Can you work these out from the model? Positions are in its coordinate system, mm. A direction names the side the tool comes from. Coordinates: 2 decimals unless noted, no trailing zeros. Write each loop counter-clockwise with the first axis right and the second up, starting at its lowest first coordinate (ties: lowest second). Pieces come first, ordered by that corner, then holes. Notation, with made-up numbers: (-25, 57.5) - (25, 57.5) arc R25 cw to (25, 71.5) - close; hole circle Ø1 at (40.5, 58). An arc over 180 degrees is marked (long way). One line per question, with ' | ' between items. Start each with the question number.
from build123d import *

# Parameters (mm, degrees)
EXTRUDE_THIN1_DEPTH     = 3
FILLET1_R               = 2
FILLET1_OF_MIRROR1_R    = 2
CIRPATTERN1_COUNT       = 2
CIRPATTERN1_ANGLE       = 90
CUT_EXTRUDE1_DEPTH      = 30.075421318
CUT_EXTRUDE1_DEPTH_BACK = 30.075421318
SKETCH3_R               = 1.625
CUT_EXTRUDE2_DEPTH      = 29.972057656
CUT_EXTRUDE2_DEPTH_BACK = 29.972057656
SKETCH4_R               = 1.5
FILLET2_R               = 8
CUT_EXTRUDE3_DEPTH      = 30.075421318
CUT_EXTRUDE3_DEPTH_BACK = 30.075421318
SKETCH5_R               = 5.5


with BuildPart() as part:
    # Sketch1 → Extrude-Thin1 (new, symmetric)
    with BuildSketch(Plane.XY):
        with BuildLine():
            Line((-20.409925586, -3), (-15.110133124, -3))
            ThreePointArc((-15.110133124, -3), (-14.249768469, -2.728728066), (-13.700594193, -2.013030215))
            Line((-13.700594193, -2.013030215), (-13.269638772, -0.828989928))
            ThreePointArc((-13.269638772, -0.828989928), (-13.08658068, -0.590423978), (-12.799792462, -0.5))
            Line((-12.799792462, -0.5), (0, -0.5))
            Line((0, -0.5), (0, 0.5))
            Line((0, 0.5), (-12.799792462, 0.5))
            ThreePointArc((-12.799792462, 0.5), (-13.660157116, 0.228728066), (-14.209331393, -0.486969785))
            Line((-14.209331393, -0.486969785), (-14.640286813, -1.671010072))
            ThreePointArc((-14.640286813, -1.671010072), (-14.823344906, -1.909576022), (-15.110133124, -2))
            Line((-15.110133124, -2), (-20.409925586, -2))
            Line((-20.409925586, -2), (-20.409925586, -3))
        make_face()
    extrude_thin1 = extrude(amount=EXTRUDE_THIN1_DEPTH, both=True)

    # Fillet1
    fillet1_edges = [part.edges().sort_by_distance(p)[0] for p in [
        (-20.409925586, -2.5, -3),
        (-20.409925586, -2.5, 3),
    ]]
    fillet(fillet1_edges, radius=FILLET1_R)

    # Mirror1: Extrude-Thin1 across plane
    add(extrude_thin1.mirror(Plane(origin=(0, 0.5, 3), x_dir=(0, 0, 1), z_dir=(1, 0, 0))))

    # Fillet1 of Mirror1
    fillet1_of_mirror1_edges = [part.edges().sort_by_distance(p)[0] for p in [
        (20.409925586, -2.5, -3),
        (20.409925586, -2.5, 3),
    ]]
    fillet(fillet1_of_mirror1_edges, radius=FILLET1_OF_MIRROR1_R)


with BuildPart() as cirpattern1_1:
    # CirPattern1: pattern copy
    add(part.part.rotate(Axis((0, 0, 0), (0, 1, 0)), 1 * CIRPATTERN1_ANGLE / (CIRPATTERN1_COUNT - 1)))


with BuildPart() as cut_extrude1_tool:
    # Sketch3 → Cut-Extrude1 (new, two sides: drawn at the far end of the back side and taken through both)
    with BuildSketch(Plane(origin=(0, 0.5, 0), x_dir=(1, 0, 0), z_dir=(0, 1, 0)).offset(-CUT_EXTRUDE1_DEPTH_BACK)):
        with Locations(Location((11.005, 0, 0), (0, 0, 270))):
            Circle(SKETCH3_R)
        with Locations(Location((0, -11.005, 0), (0, 0, 270))):
            Circle(SKETCH3_R)
        with Locations(Location((-11.005, 0, 0), (0, 0, 270))):
            Circle(SKETCH3_R)
        with Locations(Location((0, 11.005, 0), (0, 0, 270))):
            Circle(SKETCH3_R)
    extrude(amount=CUT_EXTRUDE1_DEPTH + CUT_EXTRUDE1_DEPTH_BACK)


with BuildPart() as part_1:
    add(part.part)

    # Cut-Extrude1: cut by cut_extrude1_tool
    add(cut_extrude1_tool.part, mode=Mode.SUBTRACT)


with BuildPart() as cirpattern1_1_1:
    add(cirpattern1_1.part)

    # Cut-Extrude1: cut by cut_extrude1_tool
    add(cut_extrude1_tool.part, mode=Mode.SUBTRACT)


with BuildPart() as cut_extrude2_tool:
    # Sketch4 → Cut-Extrude2 (new, two sides: drawn at the far end of the back side and taken through both)
    with BuildSketch(Plane(origin=(0, -2, 0), x_dir=(1, 0, 0), z_dir=(0, 1, 0)).offset(-CUT_EXTRUDE2_DEPTH_BACK)):
        with Locations(Location((-17.5, 0, 0), (0, 0, 180))):
            Circle(SKETCH4_R)
        with Locations(Location((0, 17.5, 0), (0, 0, 180))):
            Circle(SKETCH4_R)
        with Locations(Location((17.5, 0, 0), (0, 0, 180))):
            Circle(SKETCH4_R)
        with Locations(Location((0, -17.5, 0), (0, 0, 180))):
            Circle(SKETCH4_R)
    extrude(amount=CUT_EXTRUDE2_DEPTH + CUT_EXTRUDE2_DEPTH_BACK)


with BuildPart() as part_2:
    add(part_1.part)

    # Cut-Extrude2: cut by cut_extrude2_tool
    add(cut_extrude2_tool.part, mode=Mode.SUBTRACT)


with BuildPart() as cirpattern1_1_2:
    add(cirpattern1_1_1.part)

    # Cut-Extrude2: cut by cut_extrude2_tool
    add(cut_extrude2_tool.part, mode=Mode.SUBTRACT)


with BuildPart() as part_3:
    add(part_2.part)

    # Combine2: union CirPattern1_1
    add(cirpattern1_1_2.part)

    # Fillet2
    fillet2_edges = [part_3.edges().sort_by_distance(p)[0] for p in [
        (-3, 0, -3),
        (3, 0, -3),
        (-3, 0, 3),
        (3, 0, 3),
    ]]
    fillet(fillet2_edges, radius=FILLET2_R)

    # Sketch5 → Cut-Extrude3 (cut, two sides: drawn at the far end of the back side and taken through both)
    with BuildSketch(Plane(origin=(0, 0.5, 0), x_dir=(1, 0, 0), z_dir=(0, 1, 0)).offset(-CUT_EXTRUDE3_DEPTH_BACK)):
        with Locations(Location((0, 0, 0), (0, 0, 270))):
            Circle(SKETCH5_R)
    extrude(amount=CUT_EXTRUDE3_DEPTH + CUT_EXTRUDE3_DEPTH_BACK, mode=Mode.SUBTRACT)


solid = part_3.part
(1) If we section it at B-B on y = -2.5: List the corners of the cut face in (x, z) for me, plus the area to 3 significant figures.
(2) If we section it at D-D on x = 0: Give the number of separate pieces and of enclosed holes in the cut face, plus the area to 3 significant figures.
(3) I'm going to push flat-ended pins straight in: pin 1 (1 mm diameter, centred on y = -0.5, z = 10.5, fed in from +X); pin 2 (4 mm diameter, centred on x = 11.005, z = 0, fed in from +Y); pin 3 (6.5 mm diameter, centred on x = 0, z = 0, fed in from +Y); pin 4 (13 mm diameter, centred on x = -1, z = 4, fed in from -Y). Where does each tip first touch, or does it pass through?
(4) If I drill on probe 1 along Z at (x, y) = (17.5, -2.8); probe 2 along X at (y, z) = (-2.75, 0); probe 3 along X at (y, z) = (-0.3, 0), over which ranges is the centre line in solid material (lowest first)?
(5) If we mould it in two halves opening along X, with no side actions, what happens to faces 4 (the face through (-14.65, -2, -3)), 5 (the face through (-5.406, 0.007, 5.281)), 6 (the face through (13.49, -1.43, 0.04)), 7 (the face through (0.488, -0.007, 12.555))? For each: +X half, -X half, draft (parallel to the pull), parting line (faces both ways), or undercut.
(6) Which directions (+Z, -Z, +X, -X, +Y, -Y) give clear straight access to the entire face, cutting with the end or side of a thin tool? Please do faces 1 (the face through (14, -2, -3)), 2 (the face through (0.04, -1.43, 13.49)), 3 (the face through (-14.26, -2.736, 0.042)).
(7) If we section it at A-A on x = -17.5: List the corners of the cut face in (y, z) for me, plus the area to 3 significant figures.
(8) If we section it at C-C on z = 17.5: List the corners of the cut face in (x, y) for me, plus the area to 3 significant figures.
Values:
1) outline: (-20.41, -1) arc R2 ccw to (-18.41, -3) - (-13.99, -3) - (-13.99, 3) - (-18.41, 3) arc R2 ccw to (-20.41, 1) - close; (-3, -18.41) arc R2 ccw to (-1, -20.41) - (1, -20.41) arc R2 ccw to (3, -18.41) - (3, -13.99) - (-3, -13.99) - close; (-3, 13.99) - (3, 13.99) - (3, 18.41) arc R2 ccw to (1, 20.41) - (-1, 20.41) arc R2 ccw to (-3, 18.41) - close; (13.99, -3) - (18.41, -3) arc R2 ccw to (20.41, -1) - (20.41, 1) arc R2 ccw to (18.41, 3) - (13.99, 3) - close; hole circle Ø3 at (-17.5, 0); hole circle Ø3 at (0, -17.5); hole circle Ø3 at (0, 17.5); hole circle Ø3 at (17.5, 0) | area: 119 mm2
2) separate pieces: 6 | enclosed holes: 0 | area: 20.1 mm2
3) pin 1: x = 3.06 | pin 2: y = 0.5 | pin 3: through | pin 4: y = -0.5
4) probe 1: -3 to -1.5, 1.5 to 3 | probe 2: -20.41 to -19, -16 to -14.28, 14.28 to 16, 19 to 20.41 | probe 3: -14.13 to -12.63, -9.38 to -5.5, 5.5 to 9.38, 12.63 to 14.13
5) face 4: draft | face 5: -X half | face 6: undercut | face 7: undercut
6) face 1: -Z, +X, +Y, -Y | face 2: +X, -X, -Y | face 3: +Z, -Z, -Y
7) outline: (-3, -3) - (-2, -3) - (-2, -1.5) - (-3, -1.5) - close; (-3, 1.5) - (-2, 1.5) - (-2, 3) - (-3, 3) - close | area: 3.00 mm2
8) outline: (-3, -3) - (-1.5, -3) - (-1.5, -2) - (-3, -2) - close; (1.5, -3) - (3, -3) - (3, -2) - (1.5, -2) - close | area: 3.00 mm2
